Autodesk Inventor part; units mm, degrees
ref_plane "YZ Plane" through (0, 0, 0) normal (1, 0, 0) x (0, 1, 0)
ref_plane "XZ Plane" through (0, 0, 0) normal (0, 1, 0) x (-1, 0, 0)
ref_plane "XY Plane" through (0, 0, 0) normal (0, 0, 1) x (1, 0, 0)
sketch "Эскиз1" plane through (0, 0, 0) normal (0, 0, 1) x (1, 0, 0)
  circle A0 centre (0, 0) radius 2.1
  line L0 (-5, 14.35) -> (5, 14.35)
  line L1 (5, 14.35) -> (5, -14.35)
  line L2 (5, -14.35) -> (-5, -14.35)
  line L3 (-5, -14.35) -> (-5, 14.35)
  line L4 (-5, 14.35) -> (5, -14.35) construction
  line L5 (5, 14.35) -> (-5, -14.35) construction
  line L6 (-5, 7) -> (5, 7)
  dimension "d0" = 4.2
  dimension "d2" = 10
  dimension "d3" = 28.7
  dimension "d4" = 7
extrude "Выдавливание1" add sketch "Эскиз1" along normal blind 3.2 contours L6 L1 L2 L3
sketch "Эскиз2" plane through (0, 0, 3.2) normal (0, 0, 1) x (1, 0, 0)
  line L0 (5, -14.35) -> (5, 7)
  line L1 (5, -14.35) -> (-5, -14.35)
  line L2 (-5, -14.35) -> (-5, -11.15)
  line L3 (-5, -11.15) -> (5, -11.15)
  line L4 (5, -11.15) -> (5, -14.35)
  point P0 (0, 0)
  point P1 (5, -11.15)
  dimension "d7" = 10
  dimension "d8" = 3.2
extrude "Выдавливание2" add sketch "Эскиз2" along normal blind 13
fillet "Сопряжение1" radius 3 1 edges at (0, -11.15, 3.2)
sketch "Эскиз3" plane through (-5, -11.15, 16.2) normal (0, 1, 0) x (1, 0, 0)
  line L0 (0, 10) -> (10, 10)
  line L1 (5, 10) -> (5, 0)
  line L2 (0, 0) -> (10, 0)
  circle A0 centre (5, 5) radius 2.1
  point P0 (5, 16.2)
  dimension "d12" = 4.2
extrude "Выдавливание3" cut sketch "Эскиз3" against normal blind 13
properties part number "мертвое колесо крепл 25-26"
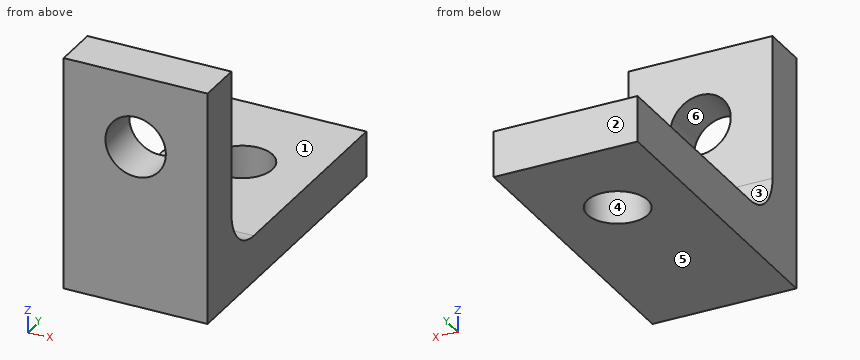
The listing builds one solid part. Answer for the finished solid, in the listing's coordinates (mm). Face numbers are marked on the shaded views. A direction names the side the tool comes from. Coordinates: 2 decimals unless noted, no trailing zeros. Write each loop counter-clockwise with the first axis right and the second up, starting at its lowest first coordinate (ties: lowest second). Pieces come first, ordered by that corner, then holes. Notation, with made-up numbers: (0.5, 60.25) -> (11.5, 60.25) arc R21 ccw to (11.5, 78.25) -> close; hole circle Ø2 at (-40, -0.5). An arc over 180 degrees is marked (long way). Write each question's results on one line, items separated by ' | '. Start each with the question number.
1) For a pull along Z with two mould halves and no side action, classify the marked faces 3, 4, 5 and 6 as +Z half, -Z half, draft (parallel to the pull), parting line (faces both ways), or undercut.
2) A flat-ended cylindrical pin translates along its axis: pin 1 Ø4 at (x, y) = (4, -2.5) entering from +Z. Find the tip coordinate at first contact, or state that the pin passes through.
3) Straight lines are drawn through the part: probe 1 along Y at (x, z) = (0, 1.9); probe 2 along X at (y, z) = (-13.35, 11.2); probe 3 along Z at (x, y) = (0, -12.7). For each, find the intervals that lie inside material, in ascending order.
4) A cutting plane is placed at C-C (z = 11.2). Determine the outline of the cut face in (x, y), then the cut area to 3 significant figures.
5) A cutting plane is placed at B-B (y = 0). Determine the outline of the cut face in (x, z).
6) A cutting plane is placed at D-D (x = 4.5). Determine the outline of the cut face in (y, z).
7) A cutting plane is placed at A-A (x = 0). Determine the outline of the cut face in (y, z).
8) A tool of negligible diameter and unlimited length cuts with its end or side. For the marked faces 1 and 2, from which of +Z, -Z, +X, -X, +Y, -Y can it reach the whole face along a straight path? Write none if from no direction.
Values follow:
1) face 3: +Z half | face 4: draft | face 5: -Z half | face 6: undercut
2) pin 1: z = 3.2
3) probe 1: -14.35 to -2.1, 2.1 to 7 | probe 2: -5 to -2.1, 2.1 to 5 | probe 3: 0 to 9.1, 13.3 to 16.2
4) outline: (-5, -14.35) -> (-2.1, -14.35) -> (-2.1, -11.15) -> (-5, -11.15) -> close; (2.1, -14.35) -> (5, -14.35) -> (5, -11.15) -> (2.1, -11.15) -> close | area: 18.6 mm²
5) outline: (-5, 0) -> (-2.1, 0) -> (-2.1, 3.2) -> (-5, 3.2) -> close; (2.1, 0) -> (5, 0) -> (5, 3.2) -> (2.1, 3.2) -> close
6) outline: (-14.35, 0) -> (7, 0) -> (7, 3.2) -> (-8.15, 3.2) arc R3 cw to (-11.15, 6.2) -> (-11.15, 16.2) -> (-14.35, 16.2) -> close
7) outline: (-14.35, 0) -> (-2.1, 0) -> (-2.1, 3.2) -> (-8.15, 3.2) arc R3 cw to (-11.15, 6.2) -> (-11.15, 9.1) -> (-14.35, 9.1) -> close; (-14.35, 13.3) -> (-11.15, 13.3) -> (-11.15, 16.2) -> (-14.35, 16.2) -> close; (2.1, 0) -> (7, 0) -> (7, 3.2) -> (2.1, 3.2) -> close
8) face 1: +Z, +X, -X, +Y | face 2: +Z, -Z, +X, -X, +Y
